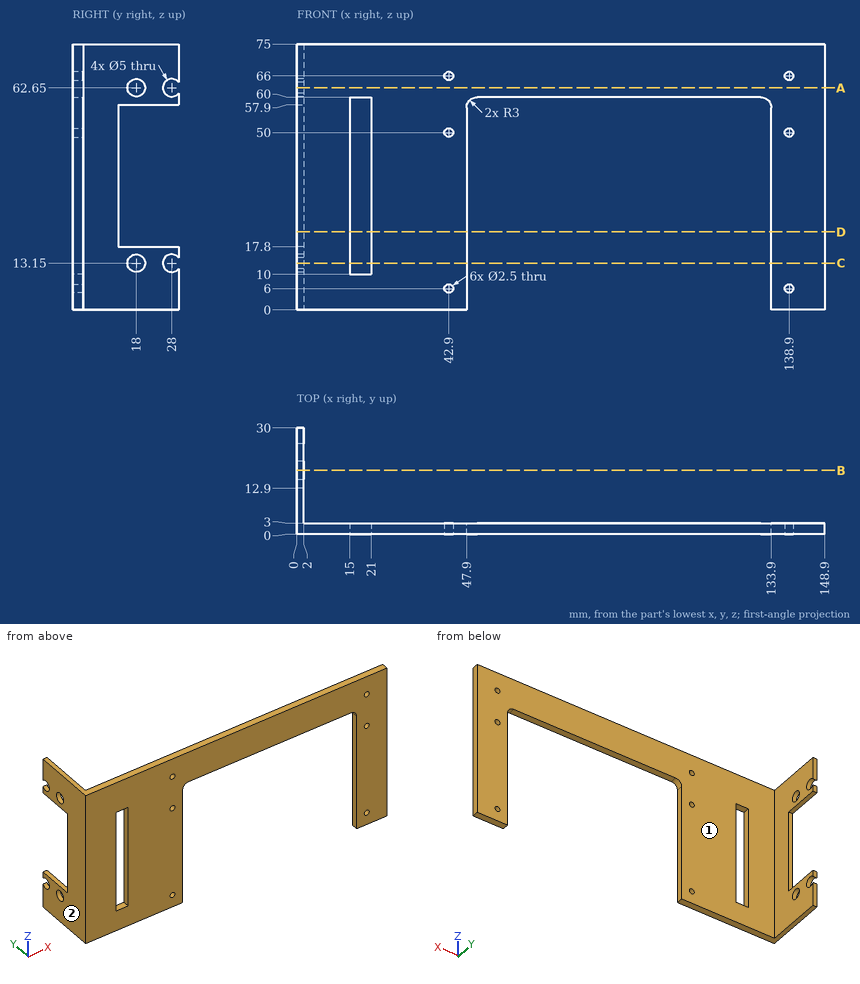
Design review of the part shown in the three views and the two pictorial views. Dimensions are in mm from the part's minimum x, y and z. A direction names the side the tool comes from. Coordinates: 2 decimals unless noted, no trailing zeros. Loops run counter-clockwise (first coordinate to the right, second up) from the corner with the lowest first, then second, coordinate; pieces in that order, holes last. Notation, with made-up numbers: (-31, 72.25) -> (1, 72.25) arc R5 ccw to (1, 81.25) -> close; hole circle Ø5 at (-31, 60). An arc over 180 degrees is marked (long way). Answer as CSV lines item,"result".
Item 1: Insertion check: pin 1 (3 mm diameter, centred on y = 28, z = 13.15, fed in from -X); pin 2 (0.6 mm diameter, centred on x = 1, y = 25.5, fed in from -Z); pin 3 (12 mm diameter, centred on x = 96, y = 8.5, fed in from -Z); pin 4 (3 mm diameter, centred on x = 138.9, z = 50, fed in from +Y). Each pin has a flat end and moves straight along its axis. Give the tip position at first contact, or say it passes through.
Results below:
pin 1,"passes through"
pin 2,"stops at z = 0"
pin 3,"stops at z = 60"
pin 4,"stops at y = 3"
Item 2: Take a section at B-B, the plane y = 18. State the section outline as (x, z) points.
Results below:
outline,"(0, 0) -> (2, 0) -> (2, 10.65) -> (0, 10.65) -> close; (0, 15.65) -> (2, 15.65) -> (2, 17.8) -> (0, 17.8) -> close; (0, 57.9) -> (2, 57.9) -> (2, 60.15) -> (0, 60.15) -> close; (0, 65.15) -> (2, 65.15) -> (2, 75) -> (0, 75) -> close"
Item 3: Take a section at C-C, the plane z = 13.15. State the section outline as (x, y) points, and give its area (3 significant figures).
Results below:
outline,"(0, 0) -> (15, 0) -> (15, 3) -> (2, 3) -> (2, 15.5) -> (0, 15.5) -> close; (0, 20.5) -> (2, 20.5) -> (2, 25.5) -> (0, 25.5) -> close; (21, 0) -> (47.9, 0) -> (47.9, 3) -> (21, 3) -> close; (133.9, 0) -> (148.9, 0) -> (148.9, 3) -> (133.9, 3) -> close"
area,"206 mm2"
Item 4: For L1, parallel to X at y = 1.5, z = 6; L2, parallel to Z at x = 0.75, y = 18; L3, parallel to X at y = 1.8, z = 66, list the stretches that pass through material, from the lowest coordinate up.
Results below:
L1,"x = 0 to 41.65, 44.15 to 47.9, 133.9 to 137.65, 140.15 to 148.9"
L2,"z = 0 to 10.65, 15.65 to 17.8, 57.9 to 60.15, 65.15 to 75"
L3,"x = 0 to 41.65, 44.15 to 137.65, 140.15 to 148.9"
Item 5: Take a section at A-A, the plane z = 62.65. State the section outline as (x, y) points, and give its area (3 significant figures).
Results below:
outline,"(0, 0) -> (148.9, 0) -> (148.9, 3) -> (2, 3) -> (2, 15.5) -> (0, 15.5) -> close; (0, 20.5) -> (2, 20.5) -> (2, 25.5) -> (0, 25.5) -> close"
area,"482 mm2"
Item 6: Take a section at D-D, the plane z = 22. State the section outline as (x, y) points.
Results below:
outline,"(0, 0) -> (15, 0) -> (15, 3) -> (2, 3) -> (2, 12.9) -> (0, 12.9) -> close; (21, 0) -> (47.9, 0) -> (47.9, 3) -> (21, 3) -> close; (133.9, 0) -> (148.9, 0) -> (148.9, 3) -> (133.9, 3) -> close"
Item 7: Machinability: for the marked faces 1 and 2, which of the approach directions +Z, -Z, +X, -X, +Y, -Y give a long, thin tool a straight path to every point of the face, cutting with its end or side? Answer none if there is none.
Results below:
face 1,"+Z, -Z, +X, +Y"
face 2,"+Z, -Z, -X, +Y, -Y"
